Read the model definition and answer for the solid it produces. Units are mm, in the model's axes. A direction names the side the tool comes from. Round coordinates to 2 decimals unless told otherwise and drop trailing zeros. Write each loop counter-clockwise with the first axis right and the second up, starting at its lowest first coordinate (ties: lowest second). Pieces come first, ordered by that corner, then holes. Notation, with made-up numbers: (-38, 36.25) - (-17, 36.25) arc R9 ccw to (-17, 52.25) - close; hole circle Ø5 at (-14.5, 4.5). An arc over 180 degrees is marked (long way). Use one line per item in the form item = value. Start each with the question number.
1) Consider line 1 along X through (y, z) = (11, 2); line 2 along Y through (x, z) = (10, 0.9); line 3 along Y through (x, z) = (5, 2.4). Determine where each line is inside the solid, lowest interval first. Write a range as from..to.
2) The part is cut by section A-A, the plane z = 0.65. Give the vertices of the cut face in (x, y).
3) Each of these flat-tipped pins is pushed along its axis until it touches: pin 1 (1.5 mm diameter, centred on x = 4, z = 2, fed in from +Y); pin 2 (1.5 mm diameter, centred on x = 20.5, z = 1.5, fed in from -Y); pin 3 (1.6 mm diameter, centred on x = 24, z = 1, fed in from -Y). Where does it stop, or does it pass through?
4) The part is cut by section B-B, the plane x = 3. Give the vertices of the cut face in (y, z), plus the area to 3 significant figures.
5) The part is cut by section D-D, the plane y = 25. Give the vertices of the cut face in (x, z).
6) For a pull along X with two mould halves and no side action, classify faces 1 (the face through (10.55, -32.494, 1.627)), 2 (the face through (-15, 20, 2)), 3 (the face through (22, 20, 2)) as released by +X, released by -X, zero draft, split by the parting line, or undercut.
7) For faces 4 (the face through (24, 30.5, 2)), 5 (the face through (35, 20, 2)), determine the directions among +Z, -Z, +X, -X, +Y, -Y from which every point of the face is accessible in a straight line to the end or side of a thin tool.
8) The part is cut by section C-C, the plane y = 44.75. Give the vertices of the cut face in (x, z), plus the area to 3 significant figures.
Autodesk Inventor part; units mm, degrees
ref_plane "YZ Plane" through (0, 0, 0) normal (1, 0, 0) x (0, 1, 0)
ref_plane "XZ Plane" through (0, 0, 0) normal (0, 1, 0) x (-1, 0, 0)
ref_plane "XY Plane" through (0, 0, 0) normal (0, 0, 1) x (1, 0, 0)
sketch "Sketch1" plane through (0, 0, 0) normal (0, 0, 1) x (1, 0, 0)
  line L0 (0, 0) -> (20, 0)
  line L1 (20, 0) -> (20, 40)
  line L2 (20, 40) -> (0, 40)
  line L3 (0, 40) -> (0, 0)
  line L4 (-15, -7.5) -> (-15, 47.5)
  line L5 (35, 47.5) -> (35, -7.5)
  arc A0 (35, 47.5) -> (-15, 47.5) centre (10, 47.5) ccw
  arc A1 (-15, -7.5) -> (35, -7.5) centre (10, -7.5) ccw
  dimension "base_servo" = 20
  dimension "altura_servo" = 40
  dimension "d2" = 15
  dimension "d3" = 15
  dimension "d4" = 55
  dimension "d5" = 55
  dimension "d9" = 7.5
extrude "Extrusion1" add sketch "Sketch1" along normal blind 3.3
sketch "Sketch2" plane through (0, 0, 3.3) normal (0, 0, 1) x (1, 0, 0)
  line L0 (22, 30.5) -> (25.3, 30.5)
  line L1 (25.3, 30.5) -> (25.3, 9.5)
  line L2 (25.3, 9.5) -> (22, 9.5)
  line L3 (22, 9.5) -> (22, 30.5)
  line L4 (-5.3, 30.5) -> (-2, 30.5)
  line L5 (-2, 30.5) -> (-2, 9.5)
  line L6 (-2, 9.5) -> (-5.3, 9.5)
  line L7 (-5.3, 9.5) -> (-5.3, 30.5)
  line L8 (0, 0) -> (0, 40)
  line L9 (20, 40) -> (20, 0)
  dimension "d12" = 3.3
  dimension "d13" = 3.3
  dimension "d14" = 21
  dimension "d16" = 9.5
  dimension "d17" = 2
  dimension "d18" = 2
extrude "Extrusion2" cut sketch "Sketch2" against normal blind 3.3
sketch "Sketch3" plane through (0, 0, 3.3) normal (0, 0, 1) x (1, 0, 0)
  circle A0 centre (5, 44.75) radius 1
  line L0 (0, 40) -> (20, 40)
  circle A1 centre (10, -4.75) radius 1
  line L1 (20, 0) -> (0, 0)
  circle A2 centre (15, 44.75) radius 1
  dimension "agujero_servo" = 2
  dimension "distancia_agujero_servo" = 4.75
  dimension "d23" = 5
  dimension "d24" = 10
  dimension "d25" = 4.75
  dimension "d28" = 4.75
  dimension "d29" = 10
extrude "Extrusion3" cut sketch "Sketch3" against normal blind 3.3 contours A0 | A1
equation "\"d3\" = d2"
equation "\"d5\" = d4"
equation "\"d9\" = 0.5 * d4 - 0.5 * altura_servo"
equation "\"d10\" = d12"
equation "\"d13\" = d12"
equation "\"d16\" = 0.5 * altura_servo - 0.5 * d14"
equation "\"d18\" = d17"
equation "\"d19\" = d12"
equation "\"d23\" = 0.25 * base_servo"
equation "\"d24\" = 0.5 * base_servo"
equation "\"d25\" = distancia_agujero_servo"
equation "\"d28\" = distancia_agujero_servo"
properties part number "soporte servo base"
Geometry results:
q1.line_1 = -15..-5.3, -2..0, 20..22, 25.3..35
q1.line_2 = -32.5..-5.75, -3.75..0, 40..72.5
q1.line_3 = -31.99..0, 40..43.75, 45.75..71.99
q2.outline = (-15, -7.5) arc R25 ccw to (35, -7.5) - (35, 47.5) arc R25 ccw to (-15, 47.5) - close; hole (-5.3, 9.5) - (-2, 9.5) - (-2, 30.5) - (-5.3, 30.5) - close; hole (0, 0) - (20, 0) - (20, 40) - (0, 40) - close; hole circle Ø2 at (5, 44.75); hole circle Ø2 at (10, -4.75); hole (22, 9.5) - (25.3, 9.5) - (25.3, 30.5) - (22, 30.5) - close
q3.pin_1 = 71.94
q3.pin_2 = -30.52
q3.pin_3 = -28.73
q4.outline = (-31.5, 0) - (0, 0) - (0, 3.3) - (-31.5, 3.3) - close; (40, 0) - (71.5, 0) - (71.5, 3.3) - (40, 3.3) - close
q4.area = 208 mm2
q5.outline = (-15, 0) - (-5.3, 0) - (-5.3, 3.3) - (-15, 3.3) - close; (-2, 0) - (0, 0) - (0, 3.3) - (-2, 3.3) - close; (20, 0) - (22, 0) - (22, 3.3) - (20, 3.3) - close; (25.3, 0) - (35, 0) - (35, 3.3) - (25.3, 3.3) - close
q6.face_1 = split by the parting line
q6.face_2 = released by -X
q6.face_3 = undercut
q7.face_4 = +Z, -Z
q7.face_5 = +Z, -Z, +X, +Y, -Y
q8.outline = (-15, 0) - (4, 0) - (4, 3.3) - (-15, 3.3) - close; (6, 0) - (35, 0) - (35, 3.3) - (6, 3.3) - close
q8.area = 158 mm2
